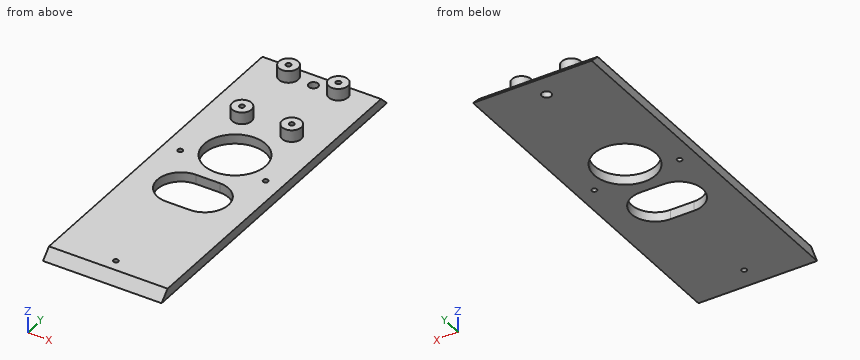
from build123d import *

# Parameters (mm, degrees)
SKETCH1_W           = 150
SKETCH1_H           = 50
BOSS_EXTRUDE1_DEPTH = 4
CHAMFER1_SIZE       = 4
SKETCH2_R           = 13
SKETCH2_R_2         = 1.065
SKETCH2_R_3         = 2
CUT_EXTRUDE2_DEPTH  = 4
SKETCH6_R           = 4.065
SKETCH6_R_2         = 1.065
BOSS_EXTRUDE2_DEPTH = 5


with BuildPart() as part:
    # Sketch1 → Boss-Extrude1 (new body)
    with BuildSketch(Plane(origin=(0, 0, 0), x_dir=(0, 1, 0), z_dir=(0, 0, 1))):
        with Locations((75, 25)):
            Rectangle(SKETCH1_W, SKETCH1_H)
    extrude(amount=BOSS_EXTRUDE1_DEPTH)

    # Chamfer1
    chamfer1_edges = [part.edges().sort_by_distance(p)[0] for p in [
        (-25, 150, 4),
        (-25, 0, 4),
    ]]
    chamfer(chamfer1_edges, length=CHAMFER1_SIZE - 0.0001)  # a hair under: the kernel refuses the full size

    # Sketch2 → Cut-Extrude2 (cut)
    with BuildSketch(Plane.XY.offset(4)):
        with Locations((-25, 88.3)):
            Circle(SKETCH2_R)
        with Locations((-25, 9)):
            Circle(SKETCH2_R_2)
        with Locations((-7, 80.3)):
            Circle(SKETCH2_R_2)
        with Locations((-43, 80.3)):
            Circle(SKETCH2_R_2)
        with Locations((-25, 140.5)):
            Circle(SKETCH2_R_3)
        with BuildLine():
            Line((-30, 70.3), (-20, 70.3))
            ThreePointArc((-20, 70.3), (-10, 60.3), (-20, 50.3))
            Line((-20, 50.3), (-30, 50.3))
            ThreePointArc((-30, 50.3), (-40, 60.3), (-30, 70.3))
        make_face()
    extrude(amount=-CUT_EXTRUDE2_DEPTH, mode=Mode.SUBTRACT)

    # Sketch6 → Boss-Extrude2 (add)
    # profile 1 of 4: a face of its own
    with BuildSketch(Plane.XY.offset(4)):
        with Locations(Location((-35.5, 140.5, 0), (0, 0, 180))):
            Circle(SKETCH6_R)
        with Locations((-35.5, 140.5)):
            Circle(SKETCH6_R_2, mode=Mode.SUBTRACT)
    # profile 2 of 4: a face of its own
    with BuildSketch(Plane.XY.offset(4)):
        with Locations(Location((-14.5, 140.5, 0), (0, 0, 180))):
            Circle(SKETCH6_R)
        with Locations((-14.5, 140.5)):
            Circle(SKETCH6_R_2, mode=Mode.SUBTRACT)
    # profile 3 of 4: a face of its own
    with BuildSketch(Plane.XY.offset(4)):
        with Locations(Location((-14.5, 109.5, 0), (0, 0, 180))):
            Circle(SKETCH6_R)
        with Locations((-14.5, 109.5)):
            Circle(SKETCH6_R_2, mode=Mode.SUBTRACT)
    # profile 4 of 4: a face of its own
    with BuildSketch(Plane.XY.offset(4)):
        with Locations(Location((-35.5, 109.5, 0), (0, 0, 180))):
            Circle(SKETCH6_R)
        with Locations((-35.5, 109.5)):
            Circle(SKETCH6_R_2, mode=Mode.SUBTRACT)
    extrude(amount=BOSS_EXTRUDE2_DEPTH)


solid = part.part
Source: CAD feature listing. Evaluate the final solid. Frame: model axes, mm. Round coordinates to 2 decimals unless told otherwise and drop trailing zeros. Loops run counter-clockwise (first coordinate to the right, second up) from the corner with the lowest first, then second, coordinate; pieces in that order, holes last. Notation, with made-up numbers: (18, 56) - (44, 56) arc R9 cw to (44, 66) - close; hole circle Ø11 at (-39.75, -10). An arc over 180 degrees is marked (long way). Write item = value, one per line. Start each with the question number.
Item 1: Section query D-D on y = 117. Output: boundary loops of the cut face in (x, z).
Item 2: First-contact query: pin 1 Ø2 at (x, y) = (-27.5, 122.5) entering from +Z; pin 2 Ø3 at (x, z) = (-36, 7) entering from -Y (3 decimals); pin 3 Ø3 at (x, z) = (-38, 3) entering from +Y. Flat tips, straight axial feed; report the tip coordinate or a pass-through.
Item 3: Section query B-B on z = 7. Output: boundary loops of the cut face in (x, y) (3 decimals), plus the area to 3 significant figures.
Item 4: Section query C-C on y = 60.3. Output: boundary loops of the cut face in (x, z).
Item 5: Section query A-A on y = 88.3. Output: boundary loops of the cut face in (x, z), plus the area to 3 significant figures.
Item 6: Material intervals for line 1 (Y direction, x = -14.5, z = 6.6) (3 decimals); line 2 (Y direction, x = -32, z = 0.75); line 3 (X direction, y = 140.5, z = 2.65), sorted ascending.
Results list:
q1.outline = (-50, 0) - (0, 0) - (0, 4) - (-50, 4) - close
q2.pin_1 = 4
q2.pin_2 = 105.435
q2.pin_3 = 148.5
q3.outline = circle Ø8.13 at (-35.5, 109.5); circle Ø8.13 at (-35.5, 140.5); circle Ø8.13 at (-14.5, 109.5); circle Ø8.13 at (-14.5, 140.5); hole circle Ø2.13 at (-35.5, 109.5); hole circle Ø2.13 at (-35.5, 140.5); hole circle Ø2.13 at (-14.5, 109.5); hole circle Ø2.13 at (-14.5, 140.5)
q3.area = 193 mm²
q4.outline = (-50, 0) - (-40, 0) - (-40, 4) - (-50, 4) - close; (-10, 0) - (0, 0) - (0, 4) - (-10, 4) - close
q5.outline = (-50, 0) - (-38, 0) - (-38, 4) - (-50, 4) - close; (-12, 0) - (0, 0) - (0, 4) - (-12, 4) - close
q5.area = 96.0 mm²
q6.line_1 = 105.435 to 108.435, 110.565 to 113.565, 136.435 to 139.435, 141.565 to 144.565
q6.line_2 = 0.75 to 50.5, 70.1 to 77.35, 99.25 to 149.25
q6.line_3 = -50 to -27, -23 to 0
